Geometry check sheet. Reference: the model listing, model coordinates, mm. Face numbers are marked on the shaded views. Round coordinates to 2 decimals unless told otherwise and drop trailing zeros. Loops run counter-clockwise (first coordinate to the right, second up) from the corner with the lowest first, then second, coordinate; pieces in that order, holes last. Notation, with made-up numbers: (30.5, 32.25) -> (64.5, 32.25) arc R21 cw to (64.5, 56.25) -> close; hole circle Ø2 at (63, 20). An arc over 180 degrees is marked (long way). Use a Markdown table: item, result. Add a question column.
Q1. Release check for a two-part mould opening along X. For the marked faces 1 and 2 record: released by +X, released by -X, zero draft, split by the parting line, or undercut.
Q2. Sectioned sample at A-A, the plane x = 43. Enter the section's corners in (y, z), then the cut area to 3 significant figures.
Q3. Material ranges on L1, parallel to Z at x = 44.5, y = 2.5; L2, parallel to Y at x = 20, z = 0.25; L3, parallel to Z at x = 27, y = 0, recorded low to high.
Q4. Sectioned sample at B-B, the plane z = -2.25. Enter the section's corners in (x, y).
Q5. Gauge pin test, flat ends, axial feed: P1, Ø1.5, axis at y = 2.5, z = -2, coming from the -X side; P2, Ø1.5, axis at x = 43.5, y = 4.5, coming from the +Z side; P3, Ø1.1, axis at x = 21, z = 1, coming from the -Y side. Record the tip position at first contact, or that the pin passes through.
Q6. Sectioned sample at C-C, the plane x = 7.5. Enter the section's corners in (y, z), then the cut area to 3 significant figures.
```python
from build123d import *

# Parameters (mm, degrees)
SKIZZE1_W                       = 53
SKIZZE1_H                       = 5
AUFSATZ_LINEAR_AUSTRAGEN1_DEPTH = 2
SKIZZE2_R                       = 1.5
AUFSATZ_LINEAR_AUSTRAGEN2_DEPTH = 4
AUFSATZ_LINEAR_AUSTRAGEN3_DEPTH = 2
SCHNITT_LINEAR_AUSTRAGEN1_DEPTH = 2
SCHNITT_LINEAR_AUSTRAGEN2_DEPTH = 62


with BuildPart() as part:
    # Skizze1 → Aufsatz-Linear austragen1 (new body)
    with BuildSketch(Plane.XY):
        with Locations((26.5, 2.5)):
            Rectangle(SKIZZE1_W, SKIZZE1_H)
    extrude(amount=AUFSATZ_LINEAR_AUSTRAGEN1_DEPTH)

    # Skizze2 → Aufsatz-Linear austragen2 (add)
    with BuildSketch(Plane(origin=(0, 0, 0), x_dir=(-1, 0, 0), z_dir=(0, 0, -1))):
        with Locations((-38, 2.5)):
            Circle(SKIZZE2_R)
        with Locations((-13, 2.5)):
            Circle(SKIZZE2_R)
    extrude(amount=AUFSATZ_LINEAR_AUSTRAGEN2_DEPTH)

    # Skizze3 → Aufsatz-Linear austragen3 (add)
    with BuildSketch(Plane.XY.offset(2)):
        with BuildLine():
            Line((9.041652249, 5.319771497), (0, 5))
            Line((0, 5), (0, 0))
            Line((0, 0), (9.041652249, -0.319771497))
            add(Edge.make_bspline(
                [(41.214812909, -0.82086692), (25.128158575, 0.571238551), (9.041652249, -0.319771497)],
                knots=[0, 0, 0, 1, 1, 1], degree=2))
            add(Edge.make_bspline(
                [(44.782995012, -1.356094236), (43.718693427, 1.301548712), (41.214812909, -0.82086692)],
                knots=[0, 0, 0, 1, 1, 1], degree=2))
            add(Edge.make_bspline(
                [(54.97075372, 2.5), (49.140580599, 2.096719237), (44.782995012, -1.356094236)],
                knots=[0, 0, 0, 1, 1, 1], degree=2))
            add(Edge.make_bspline(
                [(54.97075372, 2.5), (49.140580599, 2.903280763), (44.782995012, 6.356094236)],
                knots=[0, 0, 0, 1, 1, 1], degree=2))
            add(Edge.make_bspline(
                [(44.782995012, 6.356094236), (43.718693427, 3.698451288), (41.214812909, 5.82086692)],
                knots=[0, 0, 0, 1, 1, 1], degree=2))
            add(Edge.make_bspline(
                [(41.214812909, 5.82086692), (25.128158575, 4.428761449), (9.041652249, 5.319771497)],
                knots=[0, 0, 0, 1, 1, 1], degree=2))
        make_face()
    extrude(amount=-AUFSATZ_LINEAR_AUSTRAGEN3_DEPTH)

    # Skizze4 → Schnitt-Linear austragen1 (cut)
    with BuildSketch(Plane.XY.offset(2)):
        with BuildLine():
            Line((44.782995012, -1.356094236), (55.574942563, -1.356094236))
            Line((55.574942563, -1.356094236), (55.574942563, 6.356094236))
            Line((55.574942563, 6.356094236), (44.782995012, 6.356094236))
            add(Edge.make_bspline(
                [(44.782995012, 6.356094236), (48.809965084, 2.992691468), (54.97075372, 2.5)],
                knots=[0, 0, 0, 1, 1, 1], degree=2))
            add(Edge.make_bspline(
                [(44.782995012, -1.356094236), (48.809965084, 2.007308532), (54.97075372, 2.5)],
                knots=[0, 0, 0, 1, 1, 1], degree=2))
        make_face()
    extrude(amount=-SCHNITT_LINEAR_AUSTRAGEN1_DEPTH, mode=Mode.SUBTRACT)

    # Skizze5 → Schnitt-Linear austragen2 (cut)
    with BuildSketch(Plane.ZY):
        Polygon((1, 6.356094236), (2, 2.5), (1, -1.356094236), (2.237806681, -1.356094236), (2.319741109, 6.356094236), align=None)
    extrude(amount=-SCHNITT_LINEAR_AUSTRAGEN2_DEPTH, mode=Mode.SUBTRACT)


solid = part.part
```
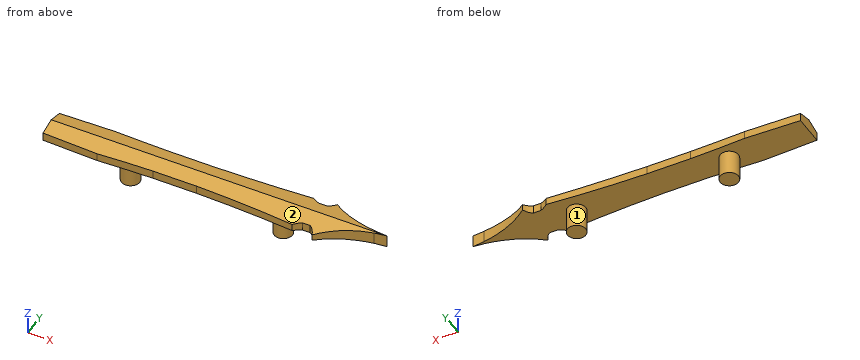
Values:
| question | item | result |
|---|---|---|
| 1 | face 1 | undercut |
| 1 | face 2 | zero draft |
| 2 | outline | (0, 0) -> (5, 0) -> (5, 1.35) -> (2.5, 2) -> (0, 1.35) -> close |
| 2 | area | 8.38 mm^2 |
| 3 | L1 | 0 to 2 |
| 3 | L2 | 0 to 5 |
| 3 | L3 | 0 to 1.35 |
| 4 | outline | circle Ø3 at (13, 2.5); circle Ø3 at (38, 2.5) |
| 5 | P1 | x = 11.5 |
| 5 | P2 | z = 1.68 |
| 5 | P3 | y = 0 |
| 6 | outline | (-0.27, 0) -> (5.27, 0) -> (5.27, 1.28) -> (2.5, 2) -> (-0.27, 1.28) -> close |
| 6 | area | 9.08 mm^2 |
